Input: part model. Units: mm. Frame: model coordinates. Face numbers are marked on the shaded views. A direction names the side the tool comes from. Coordinates: 2 decimals unless noted, no trailing zeros. Loops run counter-clockwise (first coordinate to the right, second up) from the corner with the lowest first, then second, coordinate; pieces in that order, holes last. Notation, with made-up numbers: (-18, 7) -> (-1, 7) arc R18 cw to (-1, 11) -> close; hole circle Ø8 at (6, 82). An arc over 180 degrees is marked (long way). Put each result on its own line as item: value. Start each with the question number.
1) Cut plane A-A (z = 11.5). Return the cut outline in (x, y).
2) Pull-direction query (Y, two-part tool) for the marked faces 1, 2, 3 and 4; classes: pulls with the +Y half, pulls with the -Y half, needs draft (parallel to the pull), parting line crosses it, or undercut.
3) Cut plane C-C (y = 35.5). Return the cut outline in (x, z), plus the area to 3 significant figures.
4) Material intervals for L1, parallel to X at y = -11, z = 31; L2, parallel to Y at x = 10.5, z = 12; L3, parallel to Z at x = -18, y = 27, sorted ascending.
5) Cut plane B-B (x = -23). Return the cut outline in (y, z).
6) Set-up query: the marked faces 5 and 6. Return all of +Z, -Z, +X, -X, +Y, -Y with unobstructed straight access to the full face (end or side cutting, diameter ignored); none if empty.
from build123d import *

# Parameters (mm, degrees)
F1_W     = 80
F1_H     = 170
F1_W_2   = 76
F1_H_2   = 166
F2_DEPTH = 50
F3_DEPTH = 2
F4_SIZE  = 2


with BuildPart() as f2:
    # F1 (on Top) → F2 (new body)
    with BuildSketch(Plane.XY):
        Rectangle(F1_W, F1_H)
        Rectangle(F1_W_2, F1_H_2, mode=Mode.SUBTRACT)
    extrude(amount=F2_DEPTH)

    # F1 (on Top) → F3 (join)
    with BuildSketch(Plane.XY):
        Rectangle(F1_W, F1_H)
        Rectangle(F1_W_2, F1_H_2, mode=Mode.SUBTRACT)
        Rectangle(F1_W_2, F1_H_2)
    extrude(amount=F3_DEPTH)

    # F4
    f4_edges = [f2.edges().sort_by_distance(p)[0] for p in [
        (0, 83, 2),
        (38, 0, 2),
        (-38, 0, 2),
        (0, -83, 2),
        (38, -83, 26),
        (38, 83, 26),
        (-38, 83, 26),
        (-38, -83, 26),
    ]]
    chamfer(f4_edges, length=F4_SIZE)


solid = f2.part
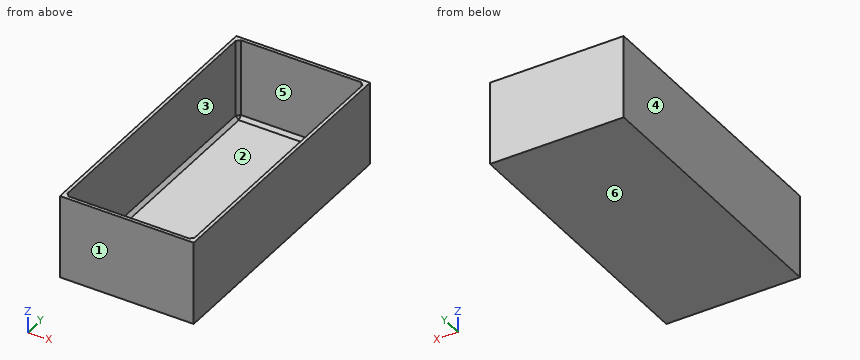
Results found:
1. outline: (-40, -85) -> (40, -85) -> (40, 85) -> (-40, 85) -> close; hole (-38, -81) -> (-36, -83) -> (36, -83) -> (38, -81) -> (38, 81) -> (36, 83) -> (-36, 83) -> (-38, 81) -> close
2. face 1: pulls with the -Y half
2. face 2: undercut
2. face 3: undercut
2. face 4: needs draft
3. outline: (-40, 0) -> (40, 0) -> (40, 50) -> (38, 50) -> (38, 4) -> (36, 2) -> (-36, 2) -> (-38, 4) -> (-38, 50) -> (-40, 50) -> close
3. area: 356 mm2
4. L1: x = -40 to -38, 38 to 40
4. L2: y = -85 to -83, 83 to 85
4. L3: z = 0 to 2
5. outline: (-85, 0) -> (85, 0) -> (85, 50) -> (83, 50) -> (83, 4) -> (81, 2) -> (-81, 2) -> (-83, 4) -> (-83, 50) -> (-85, 50) -> close
6. face 5: +Z
6. face 6: -Z, +X, -X, +Y, -Y
